Source: CAD feature listing. Evaluate the final solid. Frame: model axes, mm. A direction names the side the tool comes from. Round coordinates to 2 decimals unless told otherwise and drop trailing zeros. Loops run counter-clockwise (first coordinate to the right, second up) from the corner with the lowest first, then second, coordinate; pieces in that order, holes last. Notation, with made-up numbers: M 4.5,89 L 24.5,89 A20 ccw 24.5,112 Z; hole C 1.25,15 d6. An arc over 180 degrees is marked long. Answer as a JSON object with one key per item and string values.
from build123d import *

# Parameters (mm, degrees)
SKETCH1_W           = 126
SKETCH1_H           = 126
BOSS_EXTRUDE1_DEPTH = 5
SKETCH3_R           = 12.5
BOSS_EXTRUDE2_DEPTH = 7.5
SKETCH4_R           = 3.45
CUT_EXTRUDE1_DEPTH  = 11.5
SKETCH6_R           = 3
CUT_EXTRUDE2_DEPTH  = 179.628805068
CHAMFER1_SIZE       = 10
CHAMFER1_SIZE_2     = 7.26542528
SKETCH7_W           = 8
SKETCH7_H           = 77.91635632
BOSS_EXTRUDE3_DEPTH = 3
SKETCH8_R           = 3
CUT_EXTRUDE3_DEPTH  = 179.370401132
SKETCH9_R           = 3.45
CUT_EXTRUDE4_DEPTH  = 7
SKETCH12_W          = 78
SKETCH12_H          = 50
SKETCH12_H_2        = 38
BOSS_EXTRUDE4_DEPTH = 2
SKETCH13_W          = 72
SKETCH13_H          = 45
BOSS_EXTRUDE5_DEPTH = 1
SKETCH14_W          = 72
SKETCH14_H          = 33
BOSS_EXTRUDE6_DEPTH = 1
SKETCH17_W          = 25
SKETCH17_H          = 35
CUT_EXTRUDE6_DEPTH  = 179.370401132
SKETCH18_W          = 14
SKETCH18_H          = 20
CUT_EXTRUDE7_DEPTH  = 179.370401132
SKETCH19_R          = 3
CUT_EXTRUDE8_DEPTH  = 179.370401132


with BuildPart() as part:
    # Sketch1 → Boss-Extrude1 (new body)
    with BuildSketch(Plane(origin=(0, 0, 0), x_dir=(1, 0, 0), z_dir=(0, 1, 0))):
        with Locations((63, 63)):
            Rectangle(SKETCH1_W, SKETCH1_H)
    extrude(amount=BOSS_EXTRUDE1_DEPTH)

    # Sketch3 → Boss-Extrude2 (add)
    with BuildSketch(Plane(origin=(0, 5, 0), x_dir=(1, 0, 0), z_dir=(0, 1, 0))):
        with Locations(Location((108.6, 108.6, 0), (0, 0, 90))):
            Circle(SKETCH3_R)
    extrude(amount=BOSS_EXTRUDE2_DEPTH)

    # Sketch4 → Cut-Extrude1 (cut)
    with BuildSketch(Plane.XZ):
        with Locations(Location((108.6, -108.6, 0), (0, 0, 270))):
            Circle(SKETCH4_R)
    extrude(amount=-CUT_EXTRUDE1_DEPTH, mode=Mode.SUBTRACT)

    # Sketch6 → Cut-Extrude2 (cut, through all)
    with BuildSketch(Plane(origin=(0, 12.5, 0), x_dir=(1, 0, 0), z_dir=(0, 1, 0))):
        with Locations(Location((108.6, 108.6, 0), (0, 0, 270))):
            Circle(SKETCH6_R)
    extrude(amount=-CUT_EXTRUDE2_DEPTH, mode=Mode.SUBTRACT)

    # Chamfer1
    # the kernel refuses this chamfer: 10, 7.26542528 mm, written as the material it takes off along each edge
    with BuildSketch(Plane(origin=(108.6, 12.5, -108.6), x_dir=(0, 0, -1), z_dir=(1, 0, 0))) as chamfer1_piece_1_section:
        Polygon((12.5, -CHAMFER1_SIZE), (12.5 - CHAMFER1_SIZE_2, 0), (12.5, 0), align=None)
    chamfer1_piece_1 = revolve(axis=Axis((108.6, 12.5, -108.6), (0, 1, 0)), mode=Mode.PRIVATE)
    chamfer1_piece_1 = split(chamfer1_piece_1, bisect_by=Plane(origin=(108.6, 5, -100.650989912), z_dir=(0, 1, 0)), keep=Keep.TOP, mode=Mode.PRIVATE)
    add(chamfer1_piece_1, mode=Mode.SUBTRACT)

    # Sketch7 → Boss-Extrude3 (add)
    with BuildSketch(Plane(origin=(0, 5, 0), x_dir=(1, 0, 0), z_dir=(0, 1, 0))):
        with Locations((108.6, 48.95817816)):
            Rectangle(SKETCH7_W, SKETCH7_H)
    extrude(amount=BOSS_EXTRUDE3_DEPTH)

    # Sketch8 → Cut-Extrude3 (cut, through all)
    with BuildSketch(Plane(origin=(0, 8, 0), x_dir=(1, 0, 0), z_dir=(0, 1, 0))):
        with Locations(Location((108.6, 15, 0), (0, 0, 270))):
            Circle(SKETCH8_R)
        with Locations(Location((108.6, 31.974801407, 0), (0, 0, 270))):
            Circle(SKETCH8_R)
        with Locations(Location((108.6, 48.949602814, 0), (0, 0, 270))):
            Circle(SKETCH8_R)
        with Locations(Location((108.6, 65.924404221, 0), (0, 0, 270))):
            Circle(SKETCH8_R)
        with Locations(Location((108.6, 82.899205628, 0), (0, 0, 270))):
            Circle(SKETCH8_R)
    extrude(amount=-CUT_EXTRUDE3_DEPTH, mode=Mode.SUBTRACT)

    # Sketch9 → Cut-Extrude4 (cut)
    with BuildSketch(Plane.XZ):
        with Locations(Location((108.6, -82.899205628, 0), (0, 0, 270))):
            Circle(SKETCH9_R)
        with Locations(Location((108.6, -65.924404221, 0), (0, 0, 270))):
            Circle(SKETCH9_R)
        with Locations(Location((108.6, -48.949602814, 0), (0, 0, 270))):
            Circle(SKETCH9_R)
        with Locations(Location((108.6, -15, 0), (0, 0, 270))):
            Circle(SKETCH9_R)
        with Locations(Location((108.6, -31.974801407, 0), (0, 0, 270))):
            Circle(SKETCH9_R)
    extrude(amount=-CUT_EXTRUDE4_DEPTH, mode=Mode.SUBTRACT)

    # Sketch12 → Boss-Extrude4 (add)
    with BuildSketch(Plane(origin=(0, 5, 0), x_dir=(1, 0, 0), z_dir=(0, 1, 0))):
        with Locations((52.3, 82.899205628)):
            Rectangle(SKETCH12_W, SKETCH12_H)
        with Locations((52.3, 29.174843528)):
            Rectangle(SKETCH12_W, SKETCH12_H_2)
    extrude(amount=BOSS_EXTRUDE4_DEPTH)

    # Sketch13 → Boss-Extrude5 (add)
    with BuildSketch(Plane(origin=(0, 7, 0), x_dir=(1, 0, 0), z_dir=(0, 1, 0))):
        with Locations((52.3, 82.899205628)):
            Rectangle(SKETCH13_W, SKETCH13_H)
    extrude(amount=BOSS_EXTRUDE5_DEPTH)

    # Sketch14 → Boss-Extrude6 (add)
    with BuildSketch(Plane(origin=(0, 7, 0), x_dir=(1, 0, 0), z_dir=(0, 1, 0))):
        with Locations((52.3, 29.174843528)):
            Rectangle(SKETCH14_W, SKETCH14_H)
    extrude(amount=BOSS_EXTRUDE6_DEPTH)

    # Sketch17 → Cut-Extrude6 (cut, through all)
    with BuildSketch(Plane(origin=(0, 8, 0), x_dir=(1, 0, 0), z_dir=(0, 1, 0))):
        with Locations((52.3, 82.899205628)):
            Rectangle(SKETCH17_W, SKETCH17_H)
    extrude(amount=-CUT_EXTRUDE6_DEPTH, mode=Mode.SUBTRACT)

    # Sketch18 → Cut-Extrude7 (cut, through all)
    with BuildSketch(Plane(origin=(0, 8, 0), x_dir=(1, 0, 0), z_dir=(0, 1, 0))):
        with Locations((43.701783173, 33.658480439)):
            Rectangle(SKETCH18_W, SKETCH18_H)
        with Locations((61.019882804, 33.658480439)):
            Rectangle(SKETCH18_W, SKETCH18_H)
        with Locations((78.337982434, 33.658480439)):
            Rectangle(SKETCH18_W, SKETCH18_H)
        with Locations((26.383683543, 33.658480439)):
            Rectangle(SKETCH18_W, SKETCH18_H)
    extrude(amount=-CUT_EXTRUDE7_DEPTH, mode=Mode.SUBTRACT)

    # Sketch19 → Cut-Extrude8 (cut, through all)
    with BuildSketch(Plane(origin=(0, 8, 0), x_dir=(1, 0, 0), z_dir=(0, 1, 0))):
        with Locations(Location((26.383683543, 18.166661984, 0), (0, 0, 270))):
            Circle(SKETCH19_R)
        with Locations(Location((43.701783173, 18.166661984, 0), (0, 0, 270))):
            Circle(SKETCH19_R)
        with Locations(Location((61.019882804, 18.166661984, 0), (0, 0, 270))):
            Circle(SKETCH19_R)
        with Locations(Location((78.337982434, 18.166661984, 0), (0, 0, 270))):
            Circle(SKETCH19_R)
    extrude(amount=-CUT_EXTRUDE8_DEPTH, mode=Mode.SUBTRACT)


solid = part.part
Item 1: Section B-B on z = -25.5. Give the number of separate pieces and of enclosed holes in the cut face, then the cut area to 3 significant figures.
Answer sheet:
{"separate pieces": "5", "enclosed holes": "0", "area": "434 mm²"}
Item 2: Access query for faces 3 (the flat face through (109, 6, -87.916)), 4 (the cylindrical face through (111.51, 3.45, -84.75)), 5 (the flat face through (44, 4, -43.658)). Directions: +Z, -Z, +X, -X, +Y, -Y. A direction counts if a zero-diameter tool reaches every point of the face in a straight line with its end or side. Return the directions, or none.
Answer sheet:
{"face 3": "+X, +Y", "face 4": "-Y", "face 5": "+Y, -Y"}
Item 3: Contact query for a flat-ended pin moving along its axis: pin 1 Ø5 at (x, z) = (85, -21) entering from +Y. Output: stop coordinate, or through.
Answer sheet:
{"pin 1": "stops at y = 8"}
Item 4: Pull-direction query (Z, two-part tool) for faces 1 (the flat face through (52, 4, -100.399)), 2 (the flat face through (112, 8, -50)); classes: pulls with the +Z half, pulls with the -Z half, needs draft (parallel to the pull), parting line crosses it, or undercut.
Answer sheet:
{"face 1": "undercut", "face 2": "needs draft"}
Item 5: Section A-A on z = -82.5. Return the cut outline in (x, y), then the cut area to 3 significant figures.
Answer sheet:
{"outline": "M 0,0 L 39.8,0 L 39.8,8 L 16.3,8 L 16.3,7 L 13.3,7 L 13.3,5 L 0,5 Z; M 64.8,0 L 105.17,0 L 105.17,7 L 105.63,7 L 105.63,8 L 104.6,8 L 104.6,5 L 91.3,5 L 91.3,7 L 88.3,7 L 88.3,8 L 64.8,8 Z; M 111.57,7 L 112.03,7 L 112.03,0 L 126,0 L 126,5 L 112.6,5 L 112.6,8 L 111.57,8 Z", "area": "628 mm²"}
Item 6: Line query: probe 1 along X at (y, z) = (7.75, -87); probe 2 along X at (y, z) = (3, -28); probe 3 along Z at (x, y) = (63, 7.75). Output: solid intervals per line, ascending. Write a range as from..to.
Answer sheet:
{"probe 1": "x = 16.3..39.8, 64.8..88.3, 104.6..112.6", "probe 2": "x = 0..19.38, 33.38..36.7, 50.7..54.02, 68.02..71.34, 85.34..126", "probe 3": "z = -105.4..-100.4, -65.4..-60.4, -45.67..-43.66, -23.66..-20.42, -15.91..-12.67"}
